For this review, take the finished solid that the model builds, in its own axes (mm). Face numbers are marked on the shaded views. A direction names the side the tool comes from. Give positions to 0.01 mm unless a question says otherwise; leave off trailing zeros. Order: outer loops, then holes, each group sorted by start corner. A loop starts at its lowest first (then second) coordinate and runs counter-clockwise, first axis right, second up. Notation, with made-up numbers: (24.5, 41.25) -> (67.5, 41.25) arc R20 ccw to (67.5, 61.25) -> close; hole circle Ø11 at (31.5, -18). An arc over 180 degrees is marked (long way). One line per item, written item: value. Start each with the question number.
from build123d import *

# Parameters (mm, degrees)
F0_W     = 14.9666295471
F0_H     = 20
F4_R     = 11
F5_DEPTH = 20.001
F6_R     = 12
F6_R_2   = 9
F7_DEPTH = 3


# Not quite as in the source:
# - a pattern or mirror of a feature is missing from the dataset's text; its kind, count and spacing are read off the source's solid


with BuildPart() as f1:
    # F0 (on Front) → F1 (revolve)
    with BuildSketch(Plane.XZ):
        with Locations((7.4833147735, 0)):
            Rectangle(F0_W, F0_H)
        with BuildLine():
            ThreePointArc((14.9666295471, -10), (18, 0), (14.9666295471, 10))
            Line((14.9666295471, 10), (14.9666295471, -10))
        make_face()
    revolve(axis=Axis((0, 0, 0), (0, 0, -1)))

    # F2 (on Top) → F3 (revolve, cut)
    with BuildSketch(Plane.XY):
        Polygon((39.5, 9), (30.5, 0), (39.5, 0), align=None)
    revolve(axis=Axis((35, 0, 0), (-1, 0, 0)), mode=Mode.SUBTRACT)

    # F4 (on face) → F5 (cut, through all)
    with BuildSketch(Plane.XY.offset(10)):
        Circle(F4_R)
    extrude(amount=-F5_DEPTH, mode=Mode.SUBTRACT)

    # F6 (on Top) → F7 (join, symmetric)
    with BuildSketch(Plane.XY):
        Circle(F6_R)
        Circle(F6_R_2, mode=Mode.SUBTRACT)
    extrude(amount=F7_DEPTH, both=True)

    # F8 (on Front) → F9 (revolve, cut)
    with BuildSketch(Plane.XZ):
        Polygon((19.5, 9), (10.5, 0), (19.5, 0), align=None)
    f9 = revolve(axis=Axis((15, 0, 0), (-1, 0, 0)), mode=Mode.SUBTRACT)

    # F9_copies: F9 across plane
    add(f9.mirror(Plane(origin=(0, 0, 0), x_dir=(0, 0, -1), z_dir=(-1, 0, 0))), mode=Mode.SUBTRACT)


solid = f1.part
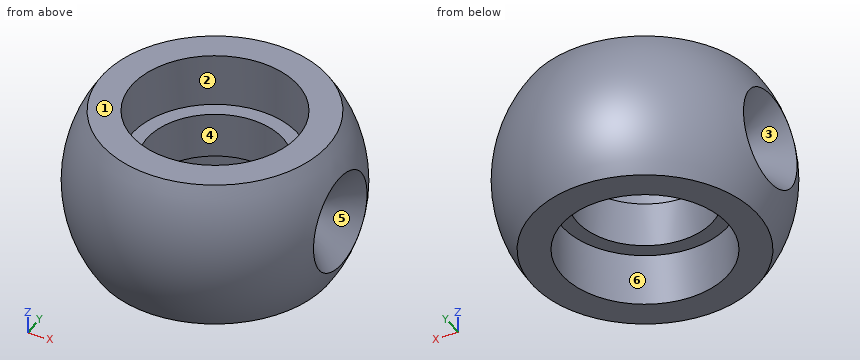
Q1. For line 1 along Y through (x, z) = (0, 0.5); line 2 along Y through (x, z) = (0, 7.25); line 3 along X through (y, z) = (9.5, -5.5), list the stretches that pass through material, from the lowest coordinate up.
Q2. Take a section at D-D (x = 2). State the section outline as (y, z) points.
Q3. Take a section at C-C (x = -10). State the section outline as (y, z) points.
Q4. Take a section at B-B (y = 10.5). State the section outline as (x, z) points.
Q5. For pin 1 Ø20 at (x, y) = (0, 0) entering from +Z; pin 2 Ø8 at (x, y) = (-4.5, 10) entering from -Z; pin 3 Ø4 at (y, z) = (-0.5, 1.5) entering from +X; pin 4 Ø2 at (y, z) = (-11, 4.5) entering from +X, all flat-tipped, find the tip position at first contact; note any pin that passes through.
Q6. For the marked faces 5 and 6, list the 3-axis set-ups (+Z, -Z, +X, -X, +Y, -Y) from which the entire face can be reached by the end or side of a thin tool; tool diameter is ignored.
Q7. Mouldability with a two-part tool opening along X and no side actions: class the marked faces 1, 2, 3 and 4 as pulls with the +X half, pulls with the -X half, needs draft (parallel to the pull), parting line crosses it, or undercut.
Q8. Take a section at A-A (x = -5). State the section outline as (y, z) points.
Answers below:
1. line 1: y = -17.99 to -9, 9 to 17.99
1. line 2: y = -16.48 to -11, 11 to 16.48
1. line 3: x = -14.27 to -5.55, 5.55 to 14.27
2. outline: (-14.83, -10) -> (-10.82, -10) -> (-10.82, -3) -> (-8.77, -3) -> (-8.77, 3) -> (-10.82, 3) -> (-10.82, 10) -> (-14.83, 10) arc R17.89 ccw to start; (8.77, -3) -> (10.82, -3) -> (10.82, -10) -> (14.83, -10) arc R17.89 ccw to (14.83, 10) -> (10.82, 10) -> (10.82, 3) -> (8.77, 3) -> close
3. outline: (-11.14, -10) -> (-4.58, -10) -> (-4.58, -3) -> (4.58, -3) -> (4.58, -10) -> (11.14, -10) arc R14.97 ccw to (11.14, 10) -> (4.58, 10) -> (4.58, 3) -> (-4.58, 3) -> (-4.58, 10) -> (-11.14, 10) arc R14.97 ccw to start
4. outline: (-10.67, -10) -> (-3.28, -10) -> (-3.28, -3) -> (3.28, -3) -> (3.28, -10) -> (10.67, -10) arc R14.62 ccw to (10.67, 10) -> (3.28, 10) -> (3.28, 3) -> (-3.28, 3) -> (-3.28, 10) -> (-10.67, 10) arc R14.62 ccw to start
5. pin 1: stops at z = 3
5. pin 2: stops at z = -10
5. pin 3: stops at x = 14.08
5. pin 4: stops at x = 14.34
6. face 5: +X
6. face 6: -Z
7. face 1: needs draft
7. face 2: undercut
7. face 3: pulls with the -X half
7. face 4: undercut
8. outline: (-14.11, -10) -> (-9.8, -10) -> (-9.8, -3) -> (-7.48, -3) -> (-7.48, 3) -> (-9.8, 3) -> (-9.8, 10) -> (-14.11, 10) arc R17.29 ccw to start; (7.48, -3) -> (9.8, -3) -> (9.8, -10) -> (14.11, -10) arc R17.29 ccw to (14.11, 10) -> (9.8, 10) -> (9.8, 3) -> (7.48, 3) -> close
